Verification items for the finished model (mm, model axes). A direction names the side the tool comes from. Give positions to 0.01 mm unless a question says otherwise; leave off trailing zeros. Order: outer loops, then holes, each group sorted by start corner. A loop starts at its lowest first (then second) coordinate and runs counter-clockwise, first axis right, second up. Notation, with made-up numbers: (-30.75, 21.5) - (-22.75, 21.5) arc R20 ccw to (-22.75, 25.5) - close; hole circle Ø6 at (32, 39.5). An arc over 180 degrees is marked (long way). Answer as a JSON object with one key per item and string values.
```python
from build123d import *

# Parameters (mm, degrees)
F0_W      = 170
F0_H      = 30
F1_DEPTH  = 60
F3_DEPTH  = 60.001
F5_DEPTH  = 60.001
F6_W      = 57.5
F6_H      = 5
F7_DEPTH  = 60.001
F8_DEPTH  = 60.001
F10_DEPTH = 6
F12_DEPTH = 6
F14_DEPTH = 30.001


with BuildPart() as f1:
    # F0 (on Front) → F1 (new body)
    with BuildSketch(Plane.XZ):
        Rectangle(F0_W, F0_H)
    extrude(amount=F1_DEPTH)

    # F2 (on face) → F3 (cut, through all)
    with BuildSketch(Plane.XZ.offset(60)):
        with BuildLine():
            Line((30, 0), (-30, 0))
            ThreePointArc((-30, 0), (-33.535534, -1.464466), (-35, -5))
            Line((-35, -5), (-35, -15))
            Line((-35, -15), (35, -15))
            Line((35, -15), (35, -5))
            ThreePointArc((35, -5), (33.535534, -1.464466), (30, 0))
        make_face()
    extrude(amount=-F3_DEPTH, mode=Mode.SUBTRACT)

    # F4 (on face) → F5 (cut, through all)
    with BuildSketch(Plane.XZ.offset(60)):
        with BuildLine():
            Line((-85, -15), (-70, -15))
            Line((-70, -15), (-70, -10))
            ThreePointArc((-70, -10), (-71.464466, -6.464466), (-75, -5))
            Line((-75, -5), (-85, -5))
            Line((-85, -5), (-85, -15))
        make_face()
        with BuildLine():
            Line((70, -10), (70, -15))
            Line((70, -15), (85, -15))
            Line((85, -15), (85, -5))
            Line((85, -5), (75, -5))
            ThreePointArc((75, -5), (71.464466, -6.464466), (70, -10))
        make_face()
    extrude(amount=-F5_DEPTH, mode=Mode.SUBTRACT)

    # F6 (on face) → F7 (cut, through all)
    with BuildSketch(Plane.XZ.offset(60)):
        with Locations((56.25, 12.5)):
            Rectangle(F6_W, F6_H)
        with Locations((-56.25, 12.5)):
            Rectangle(F6_W, F6_H)
    extrude(amount=-F7_DEPTH, mode=Mode.SUBTRACT)

    # F6 (on face) → F8 (cut, through all)
    with BuildSketch(Plane.XZ.offset(60)):
        with Locations((56.25, 12.5)):
            Rectangle(F6_W, F6_H)
        with Locations((-56.25, 12.5)):
            Rectangle(F6_W, F6_H)
    extrude(amount=-F8_DEPTH, mode=Mode.SUBTRACT)

    # F9 (on face) → F10 (join)
    with BuildSketch(Plane.XZ.offset(60)):
        with BuildLine():
            Line((27.5, 10), (85, 10))
            ThreePointArc((85, 10), (0, 36.407929), (-85, 10))
            Line((-85, 10), (-27.5, 10))
            Line((-27.5, 10), (-27.5, 15))
            Line((-27.5, 15), (27.5, 15))
            Line((27.5, 15), (27.5, 10))
        make_face()
    extrude(amount=-F10_DEPTH)

    # F11 (on face) → F12 (join)
    with BuildSketch(Plane(origin=(0, 0, 0), x_dir=(-1, 0, 0), z_dir=(0, 1, 0))):
        with BuildLine():
            Line((27.5, 10), (85, 10))
            ThreePointArc((85, 10), (0, 36.407929), (-85, 10))
            Line((-85, 10), (-27.5, 10))
            Line((-27.5, 10), (-27.5, 15))
            Line((-27.5, 15), (27.5, 15))
            Line((27.5, 15), (27.5, 10))
        make_face()
    extrude(amount=-F12_DEPTH)

    # F13 (on face) → F14 (cut, through all)
    with BuildSketch(Plane.XY.offset(15)):
        with BuildLine():
            Line((10, -20), (-10, -20))
            ThreePointArc((-10, -20), (-20, -30), (-10, -40))
            Line((-10, -40), (10, -40))
            ThreePointArc((10, -40), (20, -30), (10, -20))
        make_face()
    extrude(amount=-F14_DEPTH, mode=Mode.SUBTRACT)


solid = f1.part
```
(1) Section check C-C (y = -42). Record the cut outline in (x, z).
Computed values:
{"outline": "(-85, -5) - (-75, -5) arc R5 cw to (-70, -10) - (-70, -15) - (-35, -15) - (-35, -5) arc R5 cw to (-30, 0) - (30, 0) arc R5 cw to (35, -5) - (35, -15) - (70, -15) - (70, -10) arc R5 cw to (75, -5) - (85, -5) - (85, 10) - (27.5, 10) - (27.5, 15) - (-27.5, 15) - (-27.5, 10) - (-85, 10) - close"}
(2) Section check D-D (x = 45). Record the cut outline in (y, z), then the cut area to 3 significant figures.
Computed values:
{"outline": "(-60, -15) - (0, -15) - (0, 29.5) - (-6, 29.5) - (-6, 10) - (-54, 10) - (-54, 29.5) - (-60, 29.5) - close", "area": "1,730 mm²"}
(3) Release check for a two-part mould opening along X. For faces 6 (the cylindrical face through (34, -30, -2)), 7 (the flat face through (-35, -30, -10)), 8 (the flat face through (-80, -30, -5)), 9 (the cylindrical face through (-1.265, -2.958, 36.403)) record: pulls with the +X half, pulls with the -X half, needs draft (parallel to the pull), parting line crosses it, or undercut.
Computed values:
{"face 6": "undercut", "face 7": "undercut", "face 8": "needs draft", "face 9": "parting line crosses it"}
(4) Section check A-A (y = -30). Record the cut outline in (x, z), then the cut area to 3 significant figures.
Computed values:
{"outline": "(-85, -5) - (-75, -5) arc R5 cw to (-70, -10) - (-70, -15) - (-35, -15) - (-35, -5) arc R5 cw to (-30, 0) - (-20, 0) - (-20, 15) - (-27.5, 15) - (-27.5, 10) - (-85, 10) - close; (20, 0) - (30, 0) arc R5 cw to (35, -5) - (35, -15) - (70, -15) - (70, -10) arc R5 cw to (75, -5) - (85, -5) - (85, 10) - (27.5, 10) - (27.5, 15) - (20, 15) - close", "area": "2,600 mm²"}
(5) Material ranges on line 1 along Y through (x, z) = (-53, 10.5); line 2 along Z through (x, y) = (-44.5, -23); line 3 along X through (y, z) = (-32.5, 12), recorded low to high. Write a range as [from, to].
Computed values:
{"line 1": "y = [-60, -54], [-6, 0]", "line 2": "z = [-15, 10]", "line 3": "x = [-27.5, -19.68], [19.68, 27.5]"}
(6) Access from +Z, -Z, +X, -X, +Y, -Y to the whole of each face (thin tool, end or side, straight path). Record for faces 1 (the flat face through (-27.5, -30, 12)), 2 (the flat face through (56, -30, 10)), 3 (the flat face through (0, -20, 8)), 4 (the flat face through (80, -30, -5)), 5 (the cylindrical face through (-33, -30, -1)).
Computed values:
{"face 1": "+Z, -X", "face 2": "+Z, +X", "face 3": "+Z, -Z", "face 4": "-Z, +X, +Y, -Y", "face 5": "-Z, +Y, -Y"}
(7) Section check B-B (z = 6.5). Record the cut outline in (x, y), then the cut area to 3 significant figures.
Computed values:
{"outline": "(-85, -60) - (85, -60) - (85, 0) - (-85, 0) - close; hole (-10, -40) - (10, -40) arc R10 ccw to (10, -20) - (-10, -20) arc R10 ccw to start", "area": "9,490 mm²"}
(8) Gauge pin test, flat ends, axial feed: pin 1 Ø5 at (x, z) = (42.5, 0) entering from +Y; pin 2 Ø18 at (x, y) = (-3.5, -35) entering from -Z; pin 3 Ø8 at (x, y) = (62, -7) entering from +Z; pin 4 Ø1.5 at (y, z) = (-41, -11.5) entering from -X. Record the tip position at first contact, or that the pin passes through.
Computed values:
{"pin 1": "stops at y = 0", "pin 2": "stops at z = 0", "pin 3": "stops at z = 24.69", "pin 4": "stops at x = -70"}
